For this review, take the finished solid that the model builds, in its own axes (mm). A direction names the side the tool comes from. Coordinates: 2 decimals unless noted, no trailing zeros. Write each loop counter-clockwise with the first axis right and the second up, starting at its lowest first coordinate (ties: lowest second). Pieces come first, ordered by that corner, then holes.
1) We need section C-C on y = 83. Write out the cut boundary in (x, z), then the cut area to 3 significant figures.
2) To check wall thickness, follow line 1 along X through (y, z) = (86, 20); line 2 along Y through (x, z) = (-42.5, 8). State the ranges of each line that lie inside material, in increasing order.
3) Insertion check: P1, Ø8, axis at y = 85, z = 23.5, coming from the +X side; P2, Ø5, axis at x = -25.5, y = 83.5, coming from the +Z side; P3, Ø3, axis at x = -28, y = 83.5, coming from the -Z side. Each pin has a flat end and moves straight along its axis. Give the tip position at first contact, or say it passes through.
4) We need section A-A on x = -28. Write out the cut boundary in (y, z), then the cut area to 3 significant figures.
5) For faces 5 (the face through (-25, 85, 8)), 6 (the face through (-31, 85, 21)), 7 (the face through (-10, 85, 20)), list the 3-axis set-ups (+Z, -Z, +X, -X, +Y, -Y) from which the entire face can be reached by the end or side of a thin tool; tool diameter is ignored.
6) We need section D-D on x = -16. Write out the cut boundary in (y, z), then the cut area to 3 significant figures.
7) We need section B-B on z = 12. Write out the cut boundary in (x, y).
8) Mouldability with a two-part tool opening along Z and no side actions: class faces 1 (the face through (-25, 80, 6)), 2 (the face through (-25, 85, 32)), 3 (the face through (-35, 88, 20)), 4 (the face through (-29.034, 87.535, 19.479)) as pulls with the +Z half, pulls with the -Z half, needs draft (parallel to the pull), parting line crosses it, or undercut.
from build123d import *

# Parameters (mm, degrees)
SKETCH1_W           = 80
SKETCH1_H           = 50
BOSS_EXTRUDE1_DEPTH = 40
SKETCH2_W           = 30
SKETCH2_H           = 24
BOSS_EXTRUDE2_DEPTH = 10
SKETCH3_R           = 4
SKETCH3_R_2         = 2
CUT_EXTRUDE1_DEPTH  = 5


with BuildPart() as part:
    # Sketch1 → Boss-Extrude1 (new body)
    with BuildSketch(Plane(origin=(0, 0, 0), x_dir=(0, 1, 0), z_dir=(0, 0, 1))):
        with Locations((40, 25)):
            Rectangle(SKETCH1_W, SKETCH1_H)
    extrude(amount=BOSS_EXTRUDE1_DEPTH)

    # Sketch2 → Boss-Extrude2 (add)
    with BuildSketch(Plane(origin=(0, 80, 0), x_dir=(-1, 0, 0), z_dir=(0, 1, 0))):
        with Locations((25, 20)):
            Rectangle(SKETCH2_W, SKETCH2_H)
    extrude(amount=BOSS_EXTRUDE2_DEPTH)

    # Sketch3 → Cut-Extrude1 (cut)
    # profile 1 of 2: a face of its own
    with BuildSketch(Plane(origin=(0, 90, 0), x_dir=(-1, 0, 0), z_dir=(0, 1, 0))):
        with Locations(Location((17, 20, 0), (0, 0, 90))):
            Circle(SKETCH3_R)
        with Locations(Location((17, 20, 0), (0, 0, 90))):
            Circle(SKETCH3_R_2, mode=Mode.SUBTRACT)
    # profile 2 of 2: a face of its own
    with BuildSketch(Plane(origin=(0, 90, 0), x_dir=(-1, 0, 0), z_dir=(0, 1, 0))):
        with Locations(Location((33, 20, 0), (0, 0, 90))):
            Circle(SKETCH3_R)
        with Locations(Location((33, 20, 0), (0, 0, 90))):
            Circle(SKETCH3_R_2, mode=Mode.SUBTRACT)
    extrude(amount=-CUT_EXTRUDE1_DEPTH, mode=Mode.SUBTRACT)


solid = part.part
Result:
1. outline: (-40, 8) - (-10, 8) - (-10, 32) - (-40, 32) - close
1. area: 720 mm2
2. line 1: x = -40 to -37, -35 to -31, -29 to -21, -19 to -15, -13 to -10
2. line 2: y = 0 to 80
3. P1: stops at x = -10
3. P2: stops at z = 32
3. P3: stops at z = 8
4. outline: (0, 0) - (80, 0) - (80, 8) - (90, 8) - (90, 32) - (80, 32) - (80, 40) - (0, 40) - close
4. area: 3,440 mm2
5. face 5: -Z, +X, -X, +Y
5. face 6: +Y
5. face 7: +Z, -Z, +X, +Y
6. outline: (0, 0) - (80, 0) - (80, 8) - (90, 8) - (90, 16.13) - (85, 16.13) - (85, 18.27) - (90, 18.27) - (90, 21.73) - (85, 21.73) - (85, 23.87) - (90, 23.87) - (90, 32) - (80, 32) - (80, 40) - (0, 40) - close
6. area: 3,420 mm2
7. outline: (-50, 0) - (0, 0) - (0, 80) - (-10, 80) - (-10, 90) - (-40, 90) - (-40, 80) - (-50, 80) - close
8. face 1: needs draft
8. face 2: pulls with the +Z half
8. face 3: undercut
8. face 4: undercut
